Autodesk Inventor part; units mm, degrees
ref_plane "YZ Plane" through (0, 0, 0) normal (1, 0, 0) x (0, 1, 0)
ref_plane "XZ Plane" through (0, 0, 0) normal (0, 1, 0) x (-1, 0, 0)
ref_plane "XY Plane" through (0, 0, 0) normal (0, 0, 1) x (1, 0, 0)
sketch "Sketch1" plane through (0, 0, 0) normal (0, 1, 0) x (-1, 0, 0)
  line L0 (-6.9968, -12.4905) -> (-6.9968, 29.5095)
  line L1 (-6.9968, 29.5095) -> (-8.4968, 29.5095)
  line L2 (-7.9968, 46.0095) -> (-7.9968, 38.5095)
  line L3 (-7.9968, 38.5095) -> (-7.9968, 46.0095)
  arc A0 (-7.9968, 46.0095) -> (-9.4968, 47.5095) centre (-9.4968, 46.0095) ccw
  arc A1 (-7.9968, 46.0095) -> (-9.4968, 47.5095) centre (-9.4968, 46.0095) ccw
  line L4 (-9.4968, 47.5095) -> (-10.4968, 47.5095)
  line L5 (-9.4968, 47.5095) -> (-10.4968, 47.5095)
  line L6 (-11.9968, 46.0095) -> (-11.9968, 32.0095)
  arc A2 (-10.4968, 47.5095) -> (-11.9968, 46.0095) centre (-10.4968, 46.0095) ccw
  arc A3 (-11.9968, 32.0095) -> (-8.4968, 28.5095) centre (-8.4968, 32.0095) ccw
  line L7 (-11.9968, 46.0095) -> (-11.9968, 32.0095)
  arc A4 (-10.9968, 32.0095) -> (-8.4968, 29.5095) centre (-7.6108, 32.8955) ccw
  line L8 (-7.9968, 28.5095) -> (-7.9968, -12.4905)
  line L9 (-7.9968, 28.5095) -> (-8.4968, 28.5095)
  line L10 (-7.9968, 28.5095) -> (-8.4968, 28.5095)
  arc A5 (-11.9968, 32.0095) -> (-8.4968, 28.5095) centre (-8.4968, 32.0095) ccw
  line L11 (-8.4968, 28.5095) -> (-7.9968, 28.5095)
  line L12 (-7.9968, 28.5095) -> (-7.9968, -12.4905)
  arc A6 (-6.9968, -12.4905) -> (-5.8853, -13.4905) centre (-5.7634, -12.2372) ccw
  arc A7 (-7.9968, -12.4905) -> (-5.9968, -14.4905) centre (-5.9968, -12.4905) ccw
  arc A8 (-7.9968, -12.4905) -> (-5.9968, -14.4905) centre (-6.0394, -12.533) ccw
  line L13 (-5.9968, -14.4905) -> (1.5032, -14.4905)
  line L14 (1.5032, -14.4905) -> (1.5032, -16.2241)
  line L15 (-10.9968, 37.5095) -> (-10.9968, 32.0095)
  line L16 (-5.8853, -13.4905) -> (1.5032, -13.4905)
  line L17 (5.0532, -13.4905) -> (-2.0468, -13.4905)
  line L18 (-10.9968, 37.5095) -> (1.5032, 37.5095)
  line L19 (-7.9968, 38.5095) -> (1.5032, 38.5095)
  line L20 (10.0032, 29.5095) -> (11.5032, 29.5095)
  arc A9 (11.5032, 29.5095) -> (14.0032, 32.0095) centre (10.6172, 32.8955) ccw
  line L21 (14.0032, 37.5095) -> (14.0032, 32.0095)
  line L22 (14.0032, 37.5095) -> (1.5032, 37.5095)
  line L23 (11.0032, 38.5095) -> (1.5032, 38.5095)
  line L24 (11.0032, 38.5095) -> (11.0032, 46.0095)
  arc A10 (12.5032, 47.5095) -> (11.0032, 46.0095) centre (12.5032, 46.0095) ccw
  line L25 (12.5032, 47.5095) -> (13.5032, 47.5095)
  arc A11 (15.0032, 46.0095) -> (13.5032, 47.5095) centre (13.5032, 46.0095) ccw
  line L26 (15.0032, 46.0095) -> (15.0032, 32.0095)
  arc A12 (11.5032, 28.5095) -> (15.0032, 32.0095) centre (11.5032, 32.0095) ccw
  line L27 (11.0032, 28.5095) -> (11.5032, 28.5095)
  line L28 (11.0032, 28.5095) -> (11.0032, -12.4905)
  line L29 (10.0032, -12.4905) -> (10.0032, 29.5095)
  line L30 (8.8916, -13.4905) -> (1.5032, -13.4905)
  line L31 (9.0032, -14.4905) -> (1.5032, -14.4905)
  arc A13 (9.0032, -14.4905) -> (11.0032, -12.4905) centre (9.0032, -12.4905) ccw
  arc A14 (8.8916, -13.4905) -> (10.0032, -12.4905) centre (8.7697, -12.2372) ccw
  circle A15 centre (11.3532, 34.5095) radius 1.25
  circle A16 centre (11.3532, 34.5095) radius 1.25
  circle A17 centre (-8.3468, 34.5095) radius 1.25
  circle A18 centre (-8.3468, 34.5095) radius 1.25
  circle A19 centre (8.0032, -11.8434) radius 1.25
  circle A20 centre (8.0032, -11.8434) radius 1.25
  circle A21 centre (-4.9968, -11.8434) radius 1.25
  circle A22 centre (-4.9968, -11.8434) radius 1.25
  line L32 (-10.9968, 37.5095) -> (-11.9968, 37.5095)
  line L33 (14.0032, 37.5095) -> (15.0032, 37.5095)
  line L34 (15.0032, 37.5095) -> (15.0032, 46.0095)
  line L35 (-11.9968, 37.5095) -> (-11.9968, 46.0095)
  point P0 (0, 0)
  point P1 (5.0518, -13.4905)
  point P2 (-2.0454, -13.4905)
  point P3 (-2.0454, 37.5095)
  point P4 (5.0518, 37.5095)
  dimension "d11" = 2.5
  dimension "d6" = 3.5
  dimension "d7" = 1
  dimension "d8" = 1
  dimension "d9" = 3.5
  dimension "d10" = 0
extrude "Extrusion1" add sketch "Sketch1" along normal blind 2 contours A6 L16 L17 L30 A14 L29 L20 A9 L21 L33 L26 A12 L27 L28 A13 L31 L13 A7 L8 L9 A3 L6 L32 L15 A4 L1 L0 | L0 L1 A4 L15 L18 L22 L21 A9 L20 L29 A14 L30 L17 L16 A6
sketch "Sketch2" plane through (0, 0, 0) normal (0, -1, 0) x (1, 0, 0)
  line L0 (4.9968, 25.5095) -> (1.9968, 25.5095)
  line L1 (1.9968, 25.5095) -> (1.9968, 32.5095)
  line L2 (1.9968, 32.5095) -> (4.9968, 32.5095)
  line L3 (4.9968, 32.5095) -> (4.9968, 25.5095)
  line L4 (-5.0032, 25.5095) -> (-8.0032, 25.5095)
  line L5 (-8.0032, 25.5095) -> (-8.0032, 32.5095)
  line L6 (-8.0032, 32.5095) -> (-5.0032, 32.5095)
  line L7 (-5.0032, 32.5095) -> (-5.0032, 25.5095)
  line L8 (-8.8916, -13.4905) -> (5.8853, -13.4905)
  line L9 (-15.0032, 37.5095) -> (11.9968, 37.5095)
  line L10 (-11.0032, -12.4905) -> (-11.0032, 28.5095)
  point P0 (0, 0)
  point P1 (10.9968, 37.5095)
  point P2 (-14.0032, 37.5095)
  dimension "d15" = 7
  dimension "d18" = 3
  dimension "d21" = 7
  dimension "d32" = 3
  dimension "d36" = 5
  dimension "d41" = 3
extrude "Extrusion2" add sketch "Sketch2" along normal blind 8
fillet "Fillet1" radius 3 4 edges at (-6.5032, -8, 32.5095) (-6.5032, -8, 25.5095) (3.4968, -8, 32.5095) (3.4968, -8, 25.5095)
sketch "Sketch4" plane through (0, 0, 0) normal (0, -1, 0) x (1, 0, 0)
  line L0 (1.9968, 23.5095) -> (-5.0032, 23.5095)
  line L1 (-5.0032, 23.5095) -> (-5.0032, 34.5095)
  line L2 (-5.0032, 34.5095) -> (1.9968, 34.5095)
  line L3 (1.9968, 34.5095) -> (1.9968, 23.5095)
  line L4 (-5.0032, 32.5095) -> (-8.0032, 32.5095)
  line L5 (-5.0032, 25.5095) -> (-8.0032, 25.5095)
  point P0 (0, 0)
  dimension "d37" = 2
  dimension "d38" = 2
extrude "Extrusion4" cut sketch "Sketch4" against normal blind 1
sketch "Sketch5" plane through (4.9968, 0, 32.5095) normal (1, 0, 0) x (0, 0, -1)
  circle A0 centre (3.5, -4.5) radius 1.5
  line L0 (4, 0) -> (45, 0)
  line L1 (7, 0) -> (7, -5)
  line L2 (0, 0) -> (0, -5)
  point P0 (32.5095, 0)
  dimension "d42" = 3
  dimension "d43" = 4.5
  dimension "d44" = 3.5
  dimension "d45" = 3.5
extrude "Extrusion5" cut sketch "Sketch5" against normal blind 15
sketch "Sketch6" plane through (0, 0, 0) normal (0, -1, 0) x (1, 0, 0)
  line L0 (5.9968, -14.4905) -> (-9.0032, -14.4905)
  line L1 (-1.5032, -14.4905) -> (-1.5032, -0.2916)
  line L2 (-1.5032, -7.4905) -> (-6.5032, -7.4905)
  circle A0 centre (-6.5032, -7.4905) radius 1.5
  circle A1 centre (3.4968, -7.4905) radius 1.5
  point P0 (0, 0)
  dimension "d48" = 3
  dimension "d49" = 5
  dimension "d52" = 7
extrude "Extrusion6" cut sketch "Sketch6" against normal blind 3
equation "\"d6\" = d9"
equation "\"d7\" = d12"
equation "\"d8\" = d12"
equation "\"d32\" = d18"
Can you work these out from the model? Positions are in its coordinate system, mm. A direction names the side the tool comes from. Round coordinates to 2 decimals unless told otherwise and drop trailing zeros. Order: outer loops, then holes, each group sorted by start corner. A loop starts at its lowest first (then second) coordinate and runs counter-clockwise, first axis right, second up.
(1) I'm going to push flat-ended pins straight in: pin 1 (6 mm diameter, centred on x = 8.5, z = 28.5, fed in from -Y); pin 2 (3.5 mm diameter, centred on y = -4, z = 30, fed in from +X); pin 3 (2.5 mm diameter, centred on y = -4.5, z = 29.01, fed in from -X); pin 4 (0.6 mm diameter, centred on y = 1, z = 2, fed in from +X). Where does each tip first touch, or does it pass through?
Results are:
pin 1: stops at y = 0
pin 2: stops at x = 5
pin 3: passes through
pin 4: stops at x = 8
(2) If we section it at A-A (y = -4.5): Please give me the cut outline in (x, z).
Results are:
outline: (-8, 25.51) - (-5, 25.51) - (-5, 27.51) - (-8, 27.51) - close; (-8, 30.51) - (-5, 30.51) - (-5, 32.51) - (-8, 32.51) - close; (2, 25.51) - (5, 25.51) - (5, 27.51) - (2, 27.51) - close; (2, 30.51) - (5, 30.51) - (5, 32.51) - (2, 32.51) - close
(3) We'd pull the mould along Y, two halves only. Please class faces 1 (the face through (-1, 2, 12)), 2 (the face through (-6.482, -4.434, 30.508)), 3 (the face through (-11.003, 1, 8)): +Y half, -Y half, draft (parallel to the pull), parting line (faces both ways), or undercut.
Results are:
face 1: +Y half
face 2: undercut
face 3: draft
(4) If I drill on L1, parallel to X at y = -4.5, z = 31; L2, parallel to X at y = 1.5, z = 15.5; L3, parallel to Y at x = 2, z = -10.5, over which ranges is the centre line in solid material (lowest first)?
Results are:
L1: x = -8 to -5, 2 to 5
L2: x = -11 to 8
L3: y = 0 to 2
(5) On a 3-axis mill with a long thin cutter (end or side, diameter ignored), from which of +Z, -Z, +X, -X, +Y, -Y can I reach the whole of each face in a straight line? I mean faces 4 (the face through (4, -2, 25.51)), 5 (the face through (3.172, 0.986, -8.955)), 6 (the face through (1.997, -2, 29)), 7 (the face through (-8.003, -3, 28)). Say none if no direction works.
Results are:
face 4: -Z, +X, -X, -Y
face 5: +Y, -Y
face 6: -Y
face 7: +Z, -Z, -X, -Y
(6) If we section it at B-B (x = 4.25): Please give me the cut outline in (y, z), plus the area to 3 significant figures.
Results are:
outline: (-8, 28.51) arc R3 ccw to (-5, 25.51) - (0, 25.51) - (0, -6.19) - (2, -6.19) - (2, 37.51) - (0, 37.51) - (0, 32.51) - (-5, 32.51) arc R3 ccw to (-8, 29.51) - close; (0, -14.49) - (2, -14.49) - (2, -12.85) - (0, -12.85) - close; (0, -10.84) - (2, -10.84) - (2, -8.79) - (0, -8.79) - close; hole circle Ø3 at (-4.5, 29.01)
area: 140 mm2
(7) If we section it at D-D (z = 10.5): Please give me the cut outline in (x, y), plus the area to 3 significant figures.
Results are:
outline: (-11, 0) - (8, 0) - (8, 2) - (-11, 2) - close
area: 38.0 mm2
(8) If we section it at C-C (x = -3): Please give me the cut outline in (y, z), plus the area to 3 significant figures.
Results are:
outline: (0, -14.49) - (2, -14.49) - (2, 37.51) - (0, 37.51) - (0, 34.51) - (1, 34.51) - (1, 23.51) - (0, 23.51) - close
area: 93.0 mm2
